Can you work these out from the model? Positions are in its coordinate system, mm. A direction names the side the tool comes from. Round coordinates to 2 decimals unless told otherwise and drop trailing zeros. Order: outer loops, then holes, each group sorted by start corner. A loop starts at its lowest first (then second) coordinate and runs counter-clockwise, first axis right, second up. Notation, with made-up numbers: M 25,61 L 59,61 A18 ccw 59,96 Z; hole C 7.25,67 d8. An arc over 180 degrees is marked long. One line per question, with ' | ' between items.
```python
from build123d import *

# Parameters (mm, degrees)
F0_W          = 50
F0_H          = 75
F0_R          = 2.6717182094
F0_R_2        = 11.5
F1_DEPTH      = 150
F2_W          = 55
F2_H          = 136
F3_DEPTH      = 50
F3_DEPTH_BACK = 50


with BuildPart() as f1:
    # F0 (on Top) → F1 (new body)
    with BuildSketch(Plane.XY):
        Rectangle(F0_W, F0_H)
        with Locations((-15.5, -15.5)):
            Circle(F0_R, mode=Mode.SUBTRACT)
        with Locations((15.5, -15.5)):
            Circle(F0_R, mode=Mode.SUBTRACT)
        with Locations((-15.5, 15.5)):
            Circle(F0_R, mode=Mode.SUBTRACT)
        Circle(F0_R_2, mode=Mode.SUBTRACT)
        with Locations((15.5, 15.5)):
            Circle(F0_R, mode=Mode.SUBTRACT)
    extrude(amount=F1_DEPTH)

    # F2 (on Right) → F3 (cut, two sides)
    with BuildSketch(Plane.YZ) as f3_sk:
        with Locations((0, 75)):
            Rectangle(F2_W, F2_H)
    extrude(amount=-F3_DEPTH, mode=Mode.SUBTRACT)
    extrude(f3_sk.sketch, amount=F3_DEPTH_BACK, mode=Mode.SUBTRACT)


solid = f1.part
```
(1) Please list where these lines run through material, in increasing order: probe 1 along X at (y, z) = (-15.5, 147.25); probe 2 along Y at (x, z) = (-9, 15); probe 3 along Z at (x, y) = (-11.5, -24.5). Write a range as [from, to].
Final values:
probe 1: [-25, -18.17], [-12.83, 12.83], [18.17, 25] | probe 2: [-37.5, -27.5], [27.5, 37.5] | probe 3: [0, 7], [143, 150]
(2) On a 3-axis mill with a long thin cutter (end or side, diameter ignored), from which of +Z, -Z, +X, -X, +Y, -Y can I reach the whole of each face in a straight line? I mean faces 4 (the cylindrical face through (15.15, -12.85, 146.45)), 5 (the flat face through (0, -27.5, 74)). Say none if no direction works.
Final values:
face 4: +Z, -Z | face 5: +X, -X
(3) If we section it at A-A on y = 15.5: Please give me the cut outline in (x, z), plus the area to 3 significant figures.
Final values:
outline: M -25,0 L -18.17,0 L -18.17,7 L -25,7 Z; M -25,143 L -18.17,143 L -18.17,150 L -25,150 Z; M -12.83,0 L 12.83,0 L 12.83,7 L -12.83,7 Z; M -12.83,143 L 12.83,143 L 12.83,150 L -12.83,150 Z; M 18.17,0 L 25,0 L 25,7 L 18.17,7 Z; M 18.17,143 L 25,143 L 25,150 L 18.17,150 Z | area: 550 mm^2
(4) Will this pin go through, and if not, where does the flat tip stop? pin 1 Ø20.5 at (x, y) = (0, 0) entering from +Z.
Final values:
pin 1: through
(5) If we section it at B-B on y = 0: Please give me the cut outline in (x, z), plus the area to 3 significant figures.
Final values:
outline: M -25,0 L -11.5,0 L -11.5,7 L -25,7 Z; M -25,143 L -11.5,143 L -11.5,150 L -25,150 Z; M 11.5,0 L 25,0 L 25,7 L 11.5,7 Z; M 11.5,143 L 25,143 L 25,150 L 11.5,150 Z | area: 378 mm^2
(6) Thinking about a two-plate mould opening in X: for faces 1 (the flat face through (-25, -28, 80)), 2 (the cylindrical face through (15.15, 18.15, 3.45)), 3 (the flat face through (0, 37.5, 74)), which applies, released by +X, released by -X, zero draft, split by the parting line, or undercut?
Final values:
face 1: released by -X | face 2: undercut | face 3: zero draft
(7) If we section it at C-C on x = -15.5: Please give me the cut outline in (y, z), plus the area to 3 significant figures.
Final values:
outline: M -37.5,0 L -18.17,0 L -18.17,7 L -27.5,7 L -27.5,143 L -18.17,143 L -18.17,150 L -37.5,150 Z; M -12.83,0 L 12.83,0 L 12.83,7 L -12.83,7 Z; M -12.83,143 L 12.83,143 L 12.83,150 L -12.83,150 Z; M 18.17,0 L 37.5,0 L 37.5,150 L 18.17,150 L 18.17,143 L 27.5,143 L 27.5,7 L 18.17,7 Z | area: 3,620 mm^2
(8) If we section it at D-D on z = 32: Please give me the cut outline in (x, y), plus the area to 3 significant figures.
Final values:
outline: M -25,-37.5 L 25,-37.5 L 25,-27.5 L -25,-27.5 Z; M -25,27.5 L 25,27.5 L 25,37.5 L -25,37.5 Z | area: 1,000 mm^2
